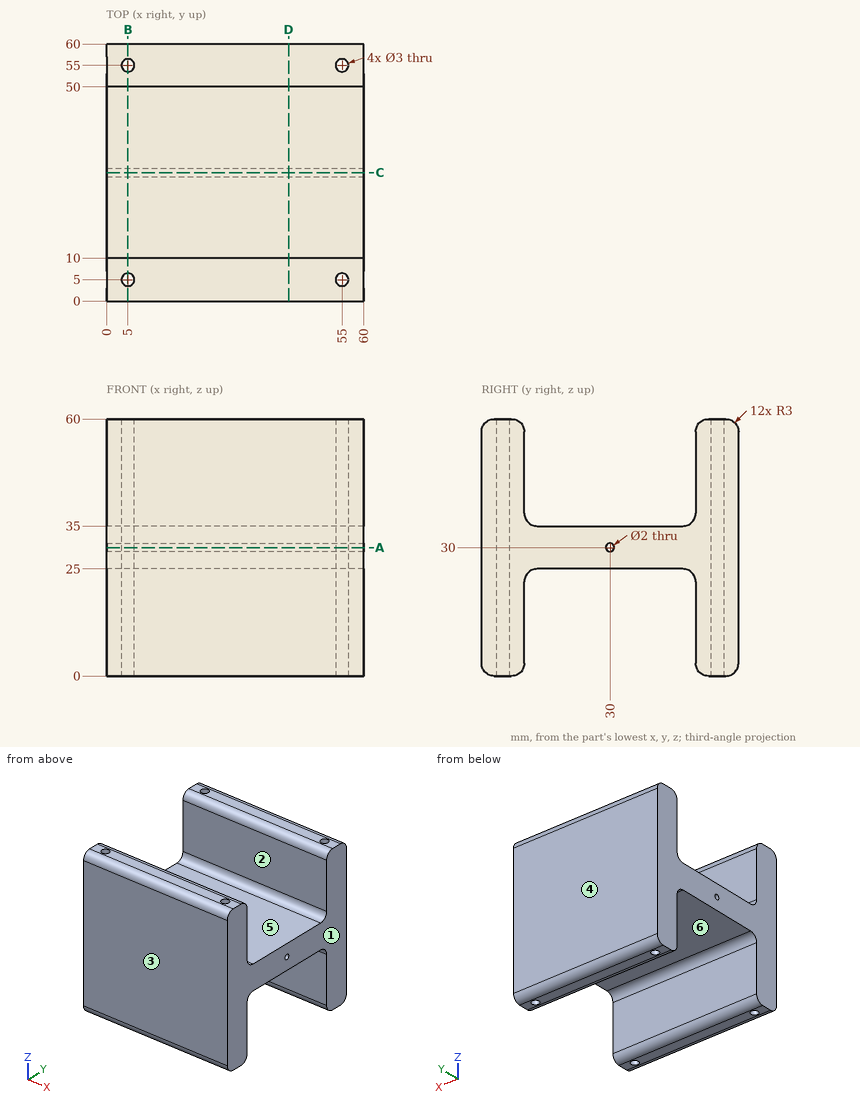
Study the drawing (mm; zero at the part's minimum x, y, z) and answer. A direction names the side the tool comes from. Give positions to 0.01 mm unless a question says otherwise; leave off trailing zeros. Order: outer loops, then holes, each group sorted by start corner. A loop starts at its lowest first (then second) coordinate and runs counter-clockwise, first axis right, second up. Notation, with made-up numbers: (-21.75, -8.5) - (27.25, -8.5) arc R17 ccw to (27.25, 18.5) - close; hole circle Ø7 at (53, 3). An arc over 180 degrees is marked (long way). Use one line per item in the form item = value. Start each with the question number.
(1) A cutting plane is placed at C-C, the plane y = 30. Write down the section's boundary in (x, z), then the cut area to 3 significant figures.
(2) Consider line 1 (Y direction, x = 55, z = 48); line 2 (Y direction, x = 23.5, z = 44); line 3 (Y direction, x = 16.5, z = 30). Determine where each line is inside the solid, lowest interval first. Write a range as from..to.
(3) A cutting plane is placed at A-A, the plane z = 30. Write down the section's boundary in (x, y), then the cut area to 3 significant figures.
(4) For the marked faces 4, 5 and 6, determine the directions among +Z, -Z, +X, -X, +Y, -Y from which every point of the face is accessible in a straight line to the end or side of a thin tool.
(5) A cutting plane is placed at B-B, the plane x = 5. State how many separate pieces and enclosed holes the cut face has, then the cut area to 3 significant figures.
(6) A cutting plane is placed at D-D, the plane x = 42.5. Write down the section's boundary in (y, z), then the cut area to 3 significant figures.
(7) The mould has two halves that part along Y. Classify the marked faces 1, 2 and 3: released by +Y, released by -Y, zero draft, split by the parting line, or undercut.
(8) Flat-ended cylindrical pins translate along their axes: pin 1 Ø4 at (x, y) = (10.5, 42.5) entering from -Z; pin 2 Ø8 at (x, y) = (9, 27.5) entering from +Z. Find the tip coordinate at first contact, or state that the pin passes through.
Ans:
q1.outline = (0, 25) - (60, 25) - (60, 29) - (0, 29) - close; (0, 31) - (60, 31) - (60, 35) - (0, 35) - close
q1.area = 480 mm^2
q2.line_1 = 0..3.5, 6.5..10, 50..53.5, 56.5..60
q2.line_2 = 0..10, 50..60
q2.line_3 = 0..29, 31..60
q3.outline = (0, 0) - (60, 0) - (60, 29) - (0, 29) - close; (0, 31) - (60, 31) - (60, 60) - (0, 60) - close; hole circle Ø3 at (5, 5); hole circle Ø3 at (5, 55); hole circle Ø3 at (55, 5); hole circle Ø3 at (55, 55)
q3.area = 3,450 mm^2
q4.face_4 = +Z, -Z, +X, -X, +Y
q4.face_5 = +Z, +X, -X
q4.face_6 = -Z, +X, -X
q5.separate_pieces = 3
q5.enclosed_holes = 1
q5.area = 1,230 mm^2
q6.outline = (0, 3) arc R3 ccw to (3, 0) - (7, 0) arc R3 ccw to (10, 3) - (10, 22) arc R3 cw to (13, 25) - (47, 25) arc R3 cw to (50, 22) - (50, 3) arc R3 ccw to (53, 0) - (57, 0) arc R3 ccw to (60, 3) - (60, 57) arc R3 ccw to (57, 60) - (53, 60) arc R3 ccw to (50, 57) - (50, 38) arc R3 cw to (47, 35) - (13, 35) arc R3 cw to (10, 38) - (10, 57) arc R3 ccw to (7, 60) - (3, 60) arc R3 ccw to (0, 57) - close; hole circle Ø2 at (30, 30)
q6.area = 1,590 mm^2
q7.face_1 = zero draft
q7.face_2 = undercut
q7.face_3 = released by -Y
q8.pin_1 = 25
q8.pin_2 = 35
